Geometry: final body of the model. Coordinates: model frame, mm. Face numbers are marked on the shaded views. A direction names the side the tool comes from. Give positions to 0.01 mm unless a question says otherwise; leave off trailing zeros. Loops run counter-clockwise (first coordinate to the right, second up) from the corner with the lowest first, then second, coordinate; pieces in that order, holes last.
```python
from build123d import *

# Parameters (mm, degrees)
F0_R     = 25
F0_R_2   = 15
F1_DEPTH = 15
F0_R_3   = 5
F2_DEPTH = 15
F0_R_4   = 10
F3_DEPTH = 15
F5_D     = 6
F6_DEPTH = 15


with BuildPart() as f1:
    # F0 (on Right) → F1 (new body, symmetric)
    with BuildSketch(Plane.YZ):
        with BuildLine():
            Line((-127.994926, -131.369472), (-120.040328, -153.224552))
            Line((-120.040328, -153.224552), (-70.040328, -153.224552))
            Line((-70.040328, -153.224552), (-64.332035, -129.30089))
            ThreePointArc((-64.332035, -129.30089), (-61.104878, -124.022259), (-55.3897, -121.652611))
            ThreePointArc((-55.3897, -121.652611), (-35.269445, -104.443983), (-45.452365, -80.004881))
            ThreePointArc((-45.452365, -80.004881), (-49.481937, -75.310092), (-49.978107, -69.143058))
            Line((-49.978107, -69.143058), (-43.121345, -40.406121))
            ThreePointArc((-43.121345, -40.406121), (-21.489193, -4.290197), (16.946071, 12.886543))
            Line((16.946071, 12.886543), (60.732447, 17.937229))
            ThreePointArc((60.732447, 17.937229), (66.796491, 16.710091), (70.977938, 12.150048))
            ThreePointArc((70.977938, 12.150048), (94.030291, -0.871109), (113.512771, 17.05637))
            ThreePointArc((113.512771, 17.05637), (116.546235, 22.448642), (122.171651, 25.024139))
            Line((122.171651, 25.024139), (184.91068, 32.260982))
            Line((184.91068, 32.260982), (137.02786, 163.817949))
            Line((137.02786, 163.817949), (-97.895296, 78.312913))
            ThreePointArc((-97.895296, 78.312913), (-151.269454, 32.618013), (-161.408791, -36.909094))
            ThreePointArc((-161.408791, -36.909094), (-162.020042, -47.608288), (-168.06693, -56.455973))
            ThreePointArc((-168.06693, -56.455973), (-178.532493, -94.846055), (-146.326766, -118.215212))
            ThreePointArc((-146.326766, -118.215212), (-135.128773, -121.960435), (-127.994926, -131.369472))
        make_face()
        with Locations((-145.518244, -83.224552)):
            Circle(F0_R, mode=Mode.SUBTRACT)
        with Locations((-57.155071, -99.221974)):
            Circle(F0_R_2, mode=Mode.SUBTRACT)
        with Locations((91.452049, 21.480684)):
            Circle(F0_R_2, mode=Mode.SUBTRACT)
    extrude(amount=F1_DEPTH, both=True)

    # F0 (on Right) → F2 (join)
    with BuildSketch(Plane.YZ):
        with Locations((91.452049, 21.480684)):
            Circle(F0_R_2)
        with Locations((91.452049, 21.480684)):
            Circle(F0_R_3, mode=Mode.SUBTRACT)
        with Locations((-57.155071, -99.221974)):
            Circle(F0_R_2)
        with Locations((-57.155071, -99.221974)):
            Circle(F0_R_3, mode=Mode.SUBTRACT)
    extrude(amount=-F2_DEPTH)

    # F0 (on Right) → F3 (join)
    with BuildSketch(Plane.YZ):
        with Locations((-145.518244, -83.224552)):
            Circle(F0_R)
        with Locations((-145.518244, -83.224552)):
            Circle(F0_R_4, mode=Mode.SUBTRACT)
    extrude(amount=-F3_DEPTH)

    # F5 (through all)
    with Locations(Plane.YZ.offset(15)):
        with Locations((123.580229, 134.979412), (138.971135, 92.693244), (154.362042, 50.407076)):
            Hole(F5_D / 2)

    # F4 (on face) → F6 (cut)
    with BuildSketch(Plane.YZ.offset(15)):
        with BuildLine():
            Line((137.02786, 163.817949), (129.980165, 161.252798))
            Line((129.980165, 161.252798), (131.277007, 157.689753))
            ThreePointArc((131.277007, 157.689753), (130.789297, 155.16595), (128.333604, 154.406337))
            ThreePointArc((128.333604, 154.406337), (103.871801, 138.38204), (121.544541, 115.083282))
            ThreePointArc((121.544541, 115.083282), (125.734082, 111.81935), (124.622722, 106.626049))
            ThreePointArc((124.622722, 106.626049), (120.177283, 85.852841), (136.935447, 72.797114))
            ThreePointArc((136.935447, 72.797114), (141.124989, 69.533182), (140.013629, 64.339881))
            ThreePointArc((140.013629, 64.339881), (141.451678, 35.132178), (170.490725, 38.580598))
            ThreePointArc((170.490725, 38.580598), (172.860165, 39.577191), (174.856042, 37.957339))
            Line((174.856042, 37.957339), (177.250928, 31.377442))
            Line((177.250928, 31.377442), (184.91068, 32.260982))
            Line((184.91068, 32.260982), (137.02786, 163.817949))
        make_face()
    extrude(amount=-F6_DEPTH, mode=Mode.SUBTRACT)


solid = f1.part
```
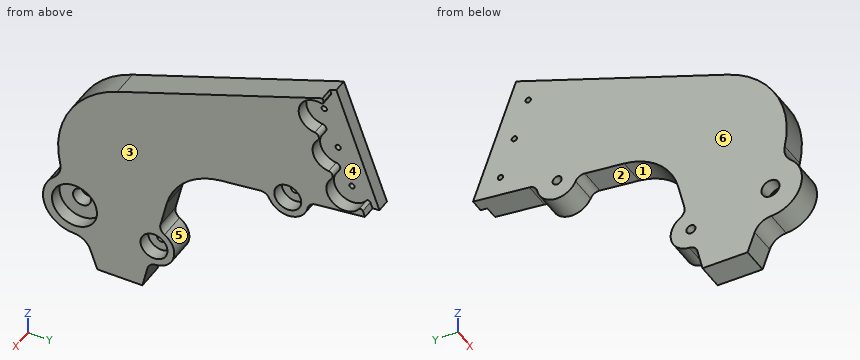
Q1. Reachability of the marked faces 1, 2 and 3 from +Z, -Z, +X, -X, +Y, -Y: full face, straight path, thin tool, end or side. Return the list, or none.
Q2. Pin query (flat end, axial travel): pin 1 Ø9 at (y, z) = (-50.5, -105) entering from +X; pin 2 Ø2 at (x, y) = (1, -2) entering from +Z; pin 3 Ø1 at (x, z) = (-1, -6) entering from +Y. Return the tip coordinate at first contact, or that it passes through.
Q3. Section query C-C, the plane y = 50. Return loops of the section in (x, z), and give its area (3 significant figures).
Q4. Section query B-B, the plane z = -5. Return loops of the section in (x, y).
Q5. Section query A-A, the plane x = -6.75. Return loops of the section in (y, z).
Q6. Mould query, pull axis X, two halves, no side actions, for the marked faces 4, 5 and 6. Classes: +X half, -X half, draft (parallel to the pull), parting line (faces both ways), or undercut.
Q7. Material intervals for probe 1 along Y at (x, z) = (-4.75, 50); probe 2 along Y at (x, z) = (-2.25, 51.5); probe 3 along Z at (x, y) = (3.5, 33.5), sorted ascending.
Resolved:
1. face 1: +X, -X
1. face 2: -Z, +X, -X
1. face 3: +Z, -Z, +X, +Y, -Y
2. pin 1: stops at x = 0
2. pin 2: stops at z = 113.58
2. pin 3: stops at y = -22.82
3. outline: (-15, 16.7) - (15, 16.7) - (15, 132.14) - (-15, 132.14) - close
3. area: 3,460 mm2
4. outline: (-15, -163.12) - (15, -163.12) - (15, -22.28) - (-15, -22.28) - close
5. outline: (-168.07, -56.46) arc R35 ccw to (-146.33, -118.22) arc R20 cw to (-127.99, -131.37) - (-120.04, -153.22) - (-70.04, -153.22) - (-64.33, -129.3) arc R10 cw to (-55.39, -121.65) arc R22.5 ccw to (-45.45, -80) arc R10 cw to (-49.98, -69.14) - (-43.12, -40.41) arc R70 cw to (16.95, 12.89) - (60.73, 17.94) arc R10 cw to (70.98, 12.15) arc R22.5 ccw to (113.51, 17.06) arc R10 cw to (122.17, 25.02) - (184.91, 32.26) - (137.03, 163.82) - (-97.9, 78.31) arc R100 ccw to (-161.41, -36.91) arc R20 cw to start; hole circle Ø20 at (-145.52, -83.22); hole circle Ø10 at (-57.16, -99.22); hole circle Ø10 at (91.45, 21.48); hole circle Ø6 at (123.58, 134.98); hole circle Ø6 at (138.97, 92.69); hole circle Ø6 at (154.36, 50.41)
6. face 4: +X half
6. face 5: draft
6. face 6: -X half
7. probe 1: y = -139.12 to 151.39, 157.33 to 178.45
7. probe 2: y = -137.79 to 151.57, 157.16 to 177.91
7. probe 3: z = 14.8 to 126.14
